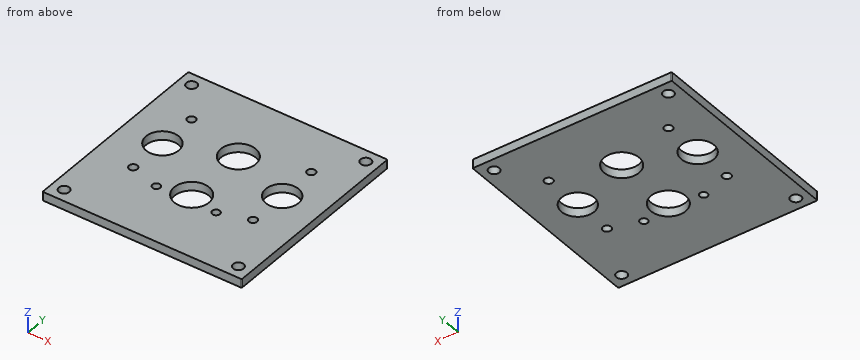
```python
from build123d import *
from build123d.topology import SkipClean

# Parameters (mm, degrees)
SKETCH1_W      = 63.5
SKETCH1_H      = 127
EXTRUDE1_DEPTH = 2.795
SKETCH2_R      = 3.3528
SKETCH2_R_2    = 10.414
SKETCH2_R_3    = 2.667
SKETCH2_R_4    = 2.4765
SKETCH2_R_5    = 11.1125
EXTRUDE2_DEPTH = 90.976375233
FILLET1_R      = 0.508


with BuildPart() as part:
    # Sketch1 → Extrude1 (new, symmetric)
    with BuildSketch(Plane.XY):
        with Locations((-31.75, 0)):
            Rectangle(SKETCH1_W, SKETCH1_H)
    extrude(amount=EXTRUDE1_DEPTH, both=True)

    # Sketch2 → Extrude2 (cut, through all)
    with BuildSketch(Plane.XY.offset(2.795)):
        with Locations((-55.5625, 55.5625)):
            Circle(SKETCH2_R)
        with Locations((-38.2016, 6.35)):
            Circle(SKETCH2_R_2)
        with Locations((-38.2082548, -19.05)):
            Circle(SKETCH2_R_3)
        with Locations((-19.05, -25.1079)):
            Circle(SKETCH2_R_4)
        with Locations((-38.2082548, 31.75)):
            Circle(SKETCH2_R_3)
        with Locations((0, -20.3454)):
            Circle(SKETCH2_R_5)
        with Locations((-55.5625, -55.5625)):
            Circle(SKETCH2_R)
        with Locations((0, 20.3454)):
            Circle(SKETCH2_R_5)
    extrude(amount=-EXTRUDE2_DEPTH, mode=Mode.SUBTRACT)

    # Fillet1
    fillet1_edges = [part.edges().sort_by_distance(p)[0] for p in [
        (-63.5, -63.5, 0),
        (-63.5, 63.5, 0),
    ]]
    fillet(fillet1_edges, radius=FILLET1_R)

    # Mirror1: part across plane


with BuildPart() as part_1:
    with SkipClean():  # the faces are left unmerged after this step: merging them gives an invalid solid
        add(part.part)
        add(part.part.mirror(Plane(origin=(0, -110.583968638, 2.795), x_dir=(0, 0, 1), z_dir=(1, 0, 0))))


solid = part_1.part
```
Part model, mm, in its own coordinate system. Give positions to 0.01 mm unless a question says otherwise; leave off trailing zeros. Loops run counter-clockwise (first coordinate to the right, second up) from the corner with the lowest first, then second, coordinate; pieces in that order, holes last. Notation, with made-up numbers: M 66,5.25 L 78,5.25 A27 cw 78,38.25 Z; hole C 58.25,58.5 d1. An arc over 180 degrees is marked long. Return JSON: item names as keys, results as strings.
1) Saw through at D-D, the plane y = -19.05. List the corners of the cut face in (x, z) (3 decimals).
Calculated:
{"outline": "M -63.5,-2.795 L -40.875,-2.795 L -40.875,2.795 L -63.5,2.795 Z; M -35.541,-2.795 L -11.037,-2.795 L -11.037,2.795 L -35.541,2.795 Z; M 11.037,-2.795 L 35.541,-2.795 L 35.541,2.795 L 11.037,2.795 Z; M 40.875,-2.795 L 63.5,-2.795 L 63.5,2.795 L 40.875,2.795 Z"}
2) Saw through at B-B, the plane y = 2. List the corners of the cut face in (x, z) (3 decimals), then the cut area to 3 significant figures.
Calculated:
{"outline": "M -63.5,-2.795 L -47.664,-2.795 L -47.664,2.795 L -63.5,2.795 Z; M -28.74,-2.795 L 28.74,-2.795 L 28.74,2.795 L -28.74,2.795 Z; M 47.664,-2.795 L 63.5,-2.795 L 63.5,2.795 L 47.664,2.795 Z", "area": "498 mm2"}
3) Drill centre lines: line 1 (Y direction, x = 0, z = -0.3); line 2 (Y direction, x = -55, z = 2.25); line 3 (X direction, y = -24.5, z = -1.85). Where is each one in solid material? Low to high.
Calculated:
{"line 1": "y = -63.5 to -31.46, -9.23 to 9.23, 31.46 to 63.5", "line 2": "y = -63.5 to -58.87, -52.26 to 52.26, 58.87 to 63.5", "line 3": "x = -63.5 to -21.45, -16.65 to -10.31, 10.31 to 16.65, 21.45 to 63.5"}
4) Saw through at C-C, the plane x = -19.05. List the corners of the cut face in (y, z) (3 decimals), then the cut area to 3 significant figures.
Calculated:
{"outline": "M -63.5,-2.795 L -27.584,-2.795 L -27.584,2.795 L -63.5,2.795 Z; M -22.631,-2.795 L 63.5,-2.795 L 63.5,2.795 L -22.631,2.795 Z", "area": "682 mm2"}
5) Saw through at A-A, the plane x = 0. List the corners of the cut face in (y, z) (3 decimals).
Calculated:
{"outline": "M -63.5,-2.795 L -31.458,-2.795 L -31.458,2.795 L -63.5,2.795 Z; M -9.233,-2.795 L 9.233,-2.795 L 9.233,2.795 L -9.233,2.795 Z; M 31.458,-2.795 L 63.5,-2.795 L 63.5,2.795 L 31.458,2.795 Z"}
